The model under review builds one solid part; all positions refer to its coordinate system, in mm. Give positions to 0.01 mm unless a question says otherwise; leave off trailing zeros. Order: outer loops, then holes, each group sorted by start corner. A loop starts at its lowest first (then second) coordinate and runs counter-clockwise, first axis right, second up. Notation, with made-up numbers: (53.25, -27) -> (78.25, -27) arc R20 cw to (78.25, 6) -> close; hole circle Ø11 at (-4, -1.75). An arc over 180 degrees is marked (long way). Use one line per item in the form item = value.
Autodesk Inventor part; units mm, degrees
ref_plane "YZ Plane" through (0, 0, 0) normal (1, 0, 0) x (0, 1, 0)
ref_plane "XZ Plane" through (0, 0, 0) normal (0, 1, 0) x (-1, 0, 0)
ref_plane "XY Plane" through (0, 0, 0) normal (0, 0, 1) x (1, 0, 0)
sketch "Sketch1" plane through (0, 0, 0) normal (1, 0, 0) x (0, 1, 0)
  line L0 (-38.1, -38.1) -> (38.1, -38.1)
  line L1 (38.1, -38.1) -> (38.1, 38.1)
  line L2 (38.1, 38.1) -> (-38.1, 38.1)
  line L3 (-38.1, 38.1) -> (-38.1, -38.1)
  line L4 (-38.1, -38.1) -> (38.1, 38.1) construction
  line L5 (38.1, -38.1) -> (-38.1, 38.1) construction
  line L6 (-41.275, 41.275) -> (41.275, 41.275)
  line L7 (41.275, 41.275) -> (41.275, -41.275)
  line L8 (41.275, -41.275) -> (-41.275, -41.275)
  line L9 (-41.275, -41.275) -> (-41.275, 41.275)
  point P0 (0, 0)
  dimension "d0" = 76.2
  dimension "d1" = 76.2
  dimension "d2" = 3.175
extrude "Extrusion1" add sketch "Sketch1" along normal blind 1.905
fillet "Fillet1" radius 0.7937 16 edges at (1.905, 0, 41.275) (0, 0, 41.275) (1.905, 0, 38.1) (0, 0, 38.1) (1.905, 0, -38.1) (0, 0, -38.1) (1.905, 0, -41.275) (0, 0, -41.275) (1.905, -38.1, 0) (0, -38.1, 0) (1.905, 38.1, 0) (1.905, 41.275, 0) (0, 38.1, 0) (0, 41.275, 0) (1.905, -41.275, 0) (0, -41.275, 0)
fillet "Fillet2" radius 3.175 12 edges at (0.9525, 41.275, 41.275) (0.2325, 41.0425, 41.0425) (1.6725, 41.0425, 41.0425) (0.9525, -41.275, 41.275) (0.2325, -41.0425, 41.0425) (1.6725, -41.0425, 41.0425) (0.9525, -41.275, -41.275) (0.2325, -41.0425, -41.0425) (1.6725, -41.0425, -41.0425) (0.9525, 41.275, -41.275) (0.2325, 41.0425, -41.0425) (1.6725, 41.0425, -41.0425)
equation "\"d0\" = 0.25 * sensorHolderFlushORingID"
equation "\"d1\" = 0.25 * sensorHolderFlushORingID"
equation "\"d2\" = oRingWidth"
equation "\"d5\" = 0.25 * oRingWidth"
equation "\"d6\" = oRingWidth"
equation "\"acrylicThickness\" = 6.35"
equation "\"height\" = 101.6"
equation "\"width\" = 101.6"
equation "\"depth\" = 101.6"
equation "\"mirrorAngle\" = 5deg"
equation "\"detectorWidth\" = 52"
equation "\"detectorHeight\" = 52"
equation "\"mirrorThickness\" = 3"
equation "\"fresnelThickness\" = 0.1"
equation "\"focalLength\" = 76.2"
equation "\"ior\" = 1.49"
equation "\"centerThickness\" = 1.524"
equation "\"fresnelAngle\" = 90deg"
equation "\"fresnelEffectiveDiameter\" = 76.2"
equation "\"mirrorSuppourtWidth\" = 38.1"
equation "\"backGrooveBit\" = 4.8006"
equation "\"sensorHolderWidth\" = 88.9"
equation "\"sensorHolderHeight\" = 88.9"
equation "\"sensorHolderSensorHeight\" = 53.975"
equation "\"sensorHolderSensorWidth\" = 53.975"
equation "\"sensorHolderORing\" = 3.175"
equation "\"sensorHolderFlushORing\" = 3.175"
equation "\"sensorHolderFlushORingID\" = 304.8"
equation "\"frontBackORingID\" = 419.1"
equation "\"oRingWidth\" = 3.175"
equation "\"sensorHolderORingID\" = 203.2"
equation "\"topBottomHorizontalMirrorGroove\" = 12.7"
equation "\"backMirrorGroove\" = 6.35"
equation "\"mirrorGroove\" = 19.05"
equation "\"mirrorGrooveFillet\" = 6.35"
equation "\"fresnelChamfer\" = 6.35"
equation "\"mirrorGrooveDrill\" = 6.35"
equation "\"mirrorGrooveMill\" = 3.175"
equation "\"fresnelMirrorChamfer\" = 6.35"
equation "\"detectorOpeningWidth\" = 76.2"
equation "\"detectorOpeningHeight\" = 76.2"
properties part number "sesnorHolderFlushORing" material "Rubber"
1. For L1, parallel to Z at x = 0.9, y = 37 (3 decimals); L2, parallel to Y at x = 1.15, z = 3; L3, parallel to Y at x = 1.8, z = 36.5, list the stretches that pass through material, from the lowest coordinate up.
Values:
L1 = -41.275 to -38.1, 38.1 to 41.275
L2 = -41.27 to -38.1, 38.1 to 41.27
L3 = -40.88 to -38.5, 38.5 to 40.88
2. Add section A-A on y = 27. Give the boundary of the cut face in (x, z) (3 decimals).
Values:
outline = (0, -40.481) arc R0.794 ccw to (0.794, -41.275) -> (1.111, -41.275) arc R0.794 ccw to (1.905, -40.481) -> (1.905, -38.894) arc R0.794 ccw to (1.111, -38.1) -> (0.794, -38.1) arc R0.794 ccw to (0, -38.894) -> close; (0, 38.894) arc R0.794 ccw to (0.794, 38.1) -> (1.111, 38.1) arc R0.794 ccw to (1.905, 38.894) -> (1.905, 40.481) arc R0.794 ccw to (1.111, 41.275) -> (0.794, 41.275) arc R0.794 ccw to (0, 40.481) -> close
3. Add section C-C on x = 0.5. Give the boundary of the cut face in (y, z).
Values:
outline = (-41.22, -38.1) arc R3.12 ccw to (-38.1, -41.22) -> (38.1, -41.22) arc R3.12 ccw to (41.22, -38.1) -> (41.22, 38.1) arc R3.12 ccw to (38.1, 41.22) -> (-38.1, 41.22) arc R3.12 ccw to (-41.22, 38.1) -> close; hole (-38.16, -38.16) -> (38.16, -38.16) -> (38.16, 38.16) -> (-38.16, 38.16) -> close
